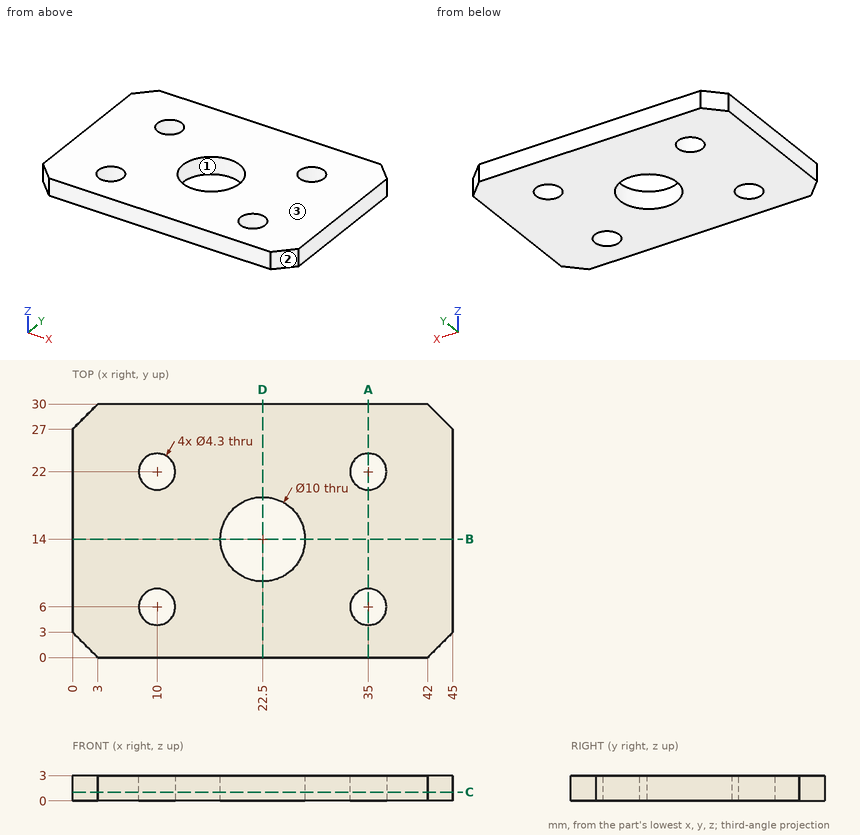
Job drawing, mm, ordinate dimensions from the low corner. One solid piece. Round coordinates to 2 decimals unless told otherwise and drop trailing zeros. Loops run counter-clockwise (first coordinate to the right, second up) from the corner with the lowest first, then second, coordinate; pieces in that order, holes last. Notation, with made-up numbers: (-7.75, 22.25) -> (19.25, 22.25) arc R25 ccw to (19.25, 47.25) -> close; hole circle Ø9 at (27.25, -24.75). An arc over 180 degrees is marked (long way). Use a Markdown table: item, result.
1) Cut at D-D, the plane x = 22.5. List the corners of the cut face in (y, z).
The answers:
| item | result |
|---|---|
| outline | (0, 0) -> (9, 0) -> (9, 3) -> (0, 3) -> close; (19, 0) -> (30, 0) -> (30, 3) -> (19, 3) -> close |
2) Cut at B-B, the plane y = 14. List the corners of the cut face in (x, z).
The answers:
| item | result |
|---|---|
| outline | (0, 0) -> (17.5, 0) -> (17.5, 3) -> (0, 3) -> close; (27.5, 0) -> (45, 0) -> (45, 3) -> (27.5, 3) -> close |
3) Pull direction X, two halves, no side cores. Call the marked faces 1, 2 and 3: pulls with the +X half, pulls with the -X half, needs draft (parallel to the pull), parting line crosses it, or undercut.
The answers:
| item | result |
|---|---|
| face 1 | undercut |
| face 2 | pulls with the +X half |
| face 3 | needs draft |
4) Cut at A-A, the plane x = 35. List the corners of the cut face in (y, z).
The answers:
| item | result |
|---|---|
| outline | (0, 0) -> (3.85, 0) -> (3.85, 3) -> (0, 3) -> close; (8.15, 0) -> (19.85, 0) -> (19.85, 3) -> (8.15, 3) -> close; (24.15, 0) -> (30, 0) -> (30, 3) -> (24.15, 3) -> close |
5) Probe line 1 (Y direction, x = 35, z = 2.35); line 2 (X direction, y = 5, z = 0.8); line 3 (Y direction, x = 22.5, z = 0.9). List the from-to ranges inside material, lowest first. Write a range as [from, to].
The answers:
| item | result |
|---|---|
| line 1 | y = [0, 3.85], [8.15, 19.85], [24.15, 30] |
| line 2 | x = [0, 8.1], [11.9, 33.1], [36.9, 45] |
| line 3 | y = [0, 9], [19, 30] |
6) Cut at C-C, the plane z = 1.05. List the corners of the cut face in (x, y).
The answers:
| item | result |
|---|---|
| outline | (0, 3) -> (3, 0) -> (42, 0) -> (45, 3) -> (45, 27) -> (42, 30) -> (3, 30) -> (0, 27) -> close; hole circle Ø4.3 at (10, 6); hole circle Ø4.3 at (10, 22); hole circle Ø10 at (22.5, 14); hole circle Ø4.3 at (35, 6); hole circle Ø4.3 at (35, 22) |
